from build123d import *

# Parameters (mm, degrees)
CROQUIS1_W              = 76.5
CROQUIS1_H              = 15.2
SALIENTE_EXTRUIR1_DEPTH = 4
CROQUIS2_W              = 70.2
CROQUIS2_H              = 3.5
CORTAR_EXTRUIR1_DEPTH   = 4
CROQUIS3_W              = 72.792072964
CROQUIS3_H              = 13.1
CORTAR_EXTRUIR2_DEPTH   = 2.5
SALIENTE_EXTRUIR2_DEPTH = 1.5


with BuildPart() as part:
    # Croquis1 → Saliente-Extruir1 (new body)
    with BuildSketch(Plane(origin=(0, 0, 0), x_dir=(1, 0, 0), z_dir=(0, 1, 0))):
        Rectangle(CROQUIS1_W, CROQUIS1_H)
    extrude(amount=SALIENTE_EXTRUIR1_DEPTH)

    # Croquis2 → Cortar-Extruir1 (cut)
    with BuildSketch(Plane(origin=(0, 4, 0), x_dir=(1, 0, 0), z_dir=(0, 1, 0))):
        with Locations((0, 3.85)):
            Rectangle(CROQUIS2_W, CROQUIS2_H)
    extrude(amount=-CORTAR_EXTRUIR1_DEPTH, mode=Mode.SUBTRACT)

    # Croquis3 → Cortar-Extruir2 (cut)
    with BuildSketch(Plane(origin=(0, 4, 0), x_dir=(1, 0, 0), z_dir=(0, 1, 0))):
        with Locations((-0.553963518, 0.15)):
            Rectangle(CROQUIS3_W, CROQUIS3_H)
    extrude(amount=-CORTAR_EXTRUIR2_DEPTH, mode=Mode.SUBTRACT)

    # Croquis4 → Saliente-Extruir2 (add)
    with BuildSketch(Plane(origin=(0, 0, 0), x_dir=(1, 0, 0), z_dir=(0, 1, 0))):
        Polygon((-12.7, -17.6), (12.7, -17.6), (38.25, -7.6), (-38.25, -7.6), align=None)
    extrude(amount=SALIENTE_EXTRUIR2_DEPTH)


solid = part.part
Geometry: final body of the model. Coordinates: model frame, mm. A direction names the side the tool comes from. Round coordinates to 2 decimals unless told otherwise and drop trailing zeros. Loops run counter-clockwise (first coordinate to the right, second up) from the corner with the lowest first, then second, coordinate; pieces in that order, holes last. Notation, with made-up numbers: M 24,-16 L 56,-16 A29 cw 56,7 Z; hole C -1.75,38.5 d7. An arc over 180 degrees is marked long. Put each result on its own line as item: value. Start each with the question number.
(1) Material intervals for line 1 along X through (y, z) = (1.9, 4.5); line 2 along Z through (x, y) = (25.5, 2.75); line 3 along X through (y, z) = (0.75, -5.5), sorted ascending. Write a range as [from, to].
(2) Draft query along Z for faces 1 (the face through (35.842, 3, 0)), 2 (the face through (0, 1, 17.6)), 3 (the face through (38.25, 2, 0)). Return one class per face: +Z half, -Z half, draft (parallel to the pull), parting line (faces both ways), or undercut.
(3) Contact query for flat-ended pins moving along their axis: pin 1 Ø0.8 at (x, y) = (14.5, 3) entering from +Z; pin 2 Ø5 at (x, z) = (26, 14.5) entering from +Y; pin 3 Ø0.8 at (x, y) = (13.5, 0.5) entering from +Z. Output: stop coordinate, or through.
(4) Section query C-C (z = 2.25). Return loops of the section in (x, y).
(5) Set-up query: faces 4 (the face through (25.3, 0.74, 12.67)), 5 (the face through (0, 1, -2.1)), 6 (the face through (-1, 3, 6.4)), 7 (the face through (-1, 3, 7.6)). Return all of +Z, -Z, +X, -X, +Y, -Y with unobstructed straight access to the full face (end or side cutting, diameter ignored); none if empty.
(6) Section query A-A (y = 3.2). Return loops of the section in (x, z), then the cut area to 3 significant figures.
(7) Section query D-D (x = -14). Return loops of the section in (y, z), then the cut area to 3 significant figures.
(8) Section query B-B (x = 1). Return loops of the section in (y, z), then the cut area to 3 significant figures.
Findings below:
1. line 1: x = [-38.25, -36.95], [35.84, 38.25]
1. line 2: z = [-7.6, -6.7], [6.4, 7.6]
1. line 3: x = [-38.25, -35.1], [35.1, 38.25]
2. face 1: undercut
2. face 2: +Z half
2. face 3: draft
3. pin 1: stops at z = 7.6
3. pin 2: stops at y = 1.5
3. pin 3: stops at z = 17.44
4. outline: M -38.25,0 L 38.25,0 L 38.25,4 L 35.84,4 L 35.84,1.5 L -36.95,1.5 L -36.95,4 L -38.25,4 Z
5. face 4: +Z, +X, +Y, -Y
5. face 5: +Y, -Y
5. face 6: +Y
5. face 7: +Z, +X, -X, +Y
6. outline: M -38.25,-7.6 L 38.25,-7.6 L 38.25,7.6 L -38.25,7.6 Z; hole M -36.95,-6.7 L 35.84,-6.7 L 35.84,6.4 L -36.95,6.4 Z
6. area: 209 mm2
7. outline: M 0,-7.6 L 4,-7.6 L 4,-6.7 L 1.5,-6.7 L 1.5,-5.6 L 0,-5.6 Z; M 0,-2.1 L 1.5,-2.1 L 1.5,6.4 L 4,6.4 L 4,7.6 L 1.5,7.6 L 1.5,17.09 L 0,17.09 Z
7. area: 37.0 mm2
8. outline: M 0,-7.6 L 4,-7.6 L 4,-6.7 L 1.5,-6.7 L 1.5,-5.6 L 0,-5.6 Z; M 0,-2.1 L 1.5,-2.1 L 1.5,6.4 L 4,6.4 L 4,7.6 L 1.5,7.6 L 1.5,17.6 L 0,17.6 Z
8. area: 37.8 mm2
